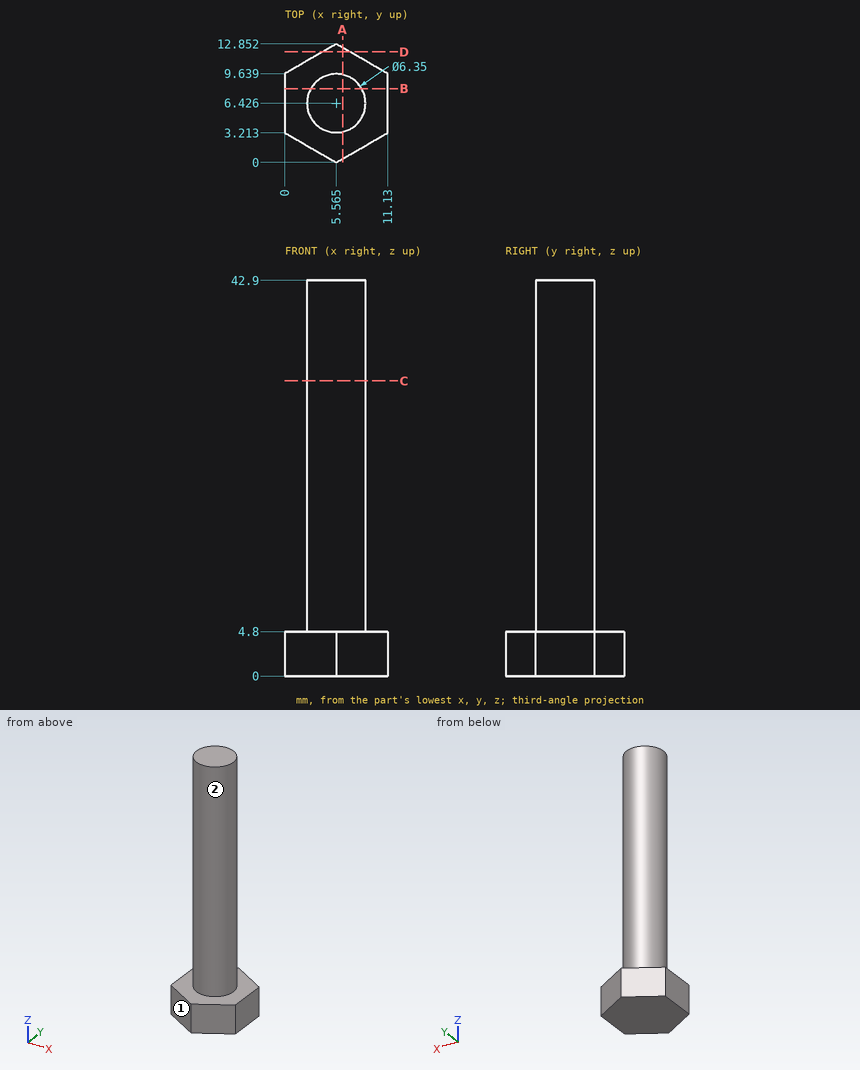
Input: dimensioned drawing with shaded views. Units: mm. Origin: part minimum x, y, z. A direction names the side the tool comes from. Round coordinates to 2 decimals unless told otherwise and drop trailing zeros. Order: outer loops, then holes, each group sorted by start corner. A loop starts at its lowest first (then second) coordinate and runs counter-clockwise, first axis right, second up. Notation, with made-up numbers: M 44.5,49 L 89.5,49 A26 cw 89.5,83 Z; hole C 78.25,38 d1. An arc over 180 degrees is marked long. Use one line per item in the form item = value. Start each with the question number.
Q1. Pin query (flat end, axial travel): pin 1 Ø6 at (x, y) = (1, 5) entering from -Z; pin 2 Ø1.5 at (y, z) = (1.5, 22) entering from -X; pin 3 Ø5 at (x, z) = (6.5, 34) entering from +Y; pin 4 Ø6 at (y, z) = (5.5, 30.5) entering from +X. Return the tip coordinate at first contact, or that it passes through.
Q2. Cut plane D-D (y = 12). Return loops of the section in (x, z), and give its area (3 significant figures).
Q3. Access query for the marked faces 1 and 2. Directions: +Z, -Z, +X, -X, +Y, -Y. A direction counts if a zero-diameter tool reaches every point of the face in a straight line with its end or side. Return the directions, or none.
Q4. Material intervals for line 1 (X direction, y = 6.25, z = 18) (1 decimal); line 2 (Z direction, x = 2, y = 6.25); line 3 (Y direction, x = 3.25, z = 34.5), sorted ascending. Write a range as [from, to].
Q5. Cut plane C-C (z = 32). Return loops of the section in (x, y) (3 decimals).
Q6. Cut plane B-B (y = 8). Return loops of the section in (x, z).
Q7. Cut plane A-A (x = 6.25). Return loops of the section in (y, z).
Geometry results:
q1.pin_1 = 0
q1.pin_2 = through
q1.pin_3 = 9.6
q1.pin_4 = 8.74
q2.outline = M 4.09,0 L 7.04,0 L 7.04,4.8 L 4.09,4.8 Z
q2.area = 14.2 mm^2
q3.face_1 = +Z, -Z, -X, -Y
q3.face_2 = +Z
q4.line_1 = [2.4, 8.7]
q4.line_2 = [0, 4.8]
q4.line_3 = [4.25, 8.6]
q5.outline = C 5.565,6.426 d6.35
q6.outline = M 0,0 L 11.13,0 L 11.13,4.8 L 8.32,4.8 L 8.32,42.9 L 2.81,42.9 L 2.81,4.8 L 0,4.8 Z
q7.outline = M 0.4,0 L 12.46,0 L 12.46,4.8 L 9.53,4.8 L 9.53,42.9 L 3.33,42.9 L 3.33,4.8 L 0.4,4.8 Z
